Could you check a few things on this drawing? It's one solid part, dimensions in mm from its lowest x, y, z. A direction names the side the tool comes from. Round coordinates to 2 decimals unless told otherwise and drop trailing zeros. Write each loop counter-clockwise with the first axis right and the second up, starting at its lowest first coordinate (ties: lowest second). Pieces come first, ordered by that corner, then holes. Notation, with made-up numbers: (57, 81.25) -> (99, 81.25) arc R27 cw to (99, 108.25) -> close; hole circle Ø11 at (38.5, 54). An arc over 180 degrees is marked (long way). Answer as CSV lines item,"result".
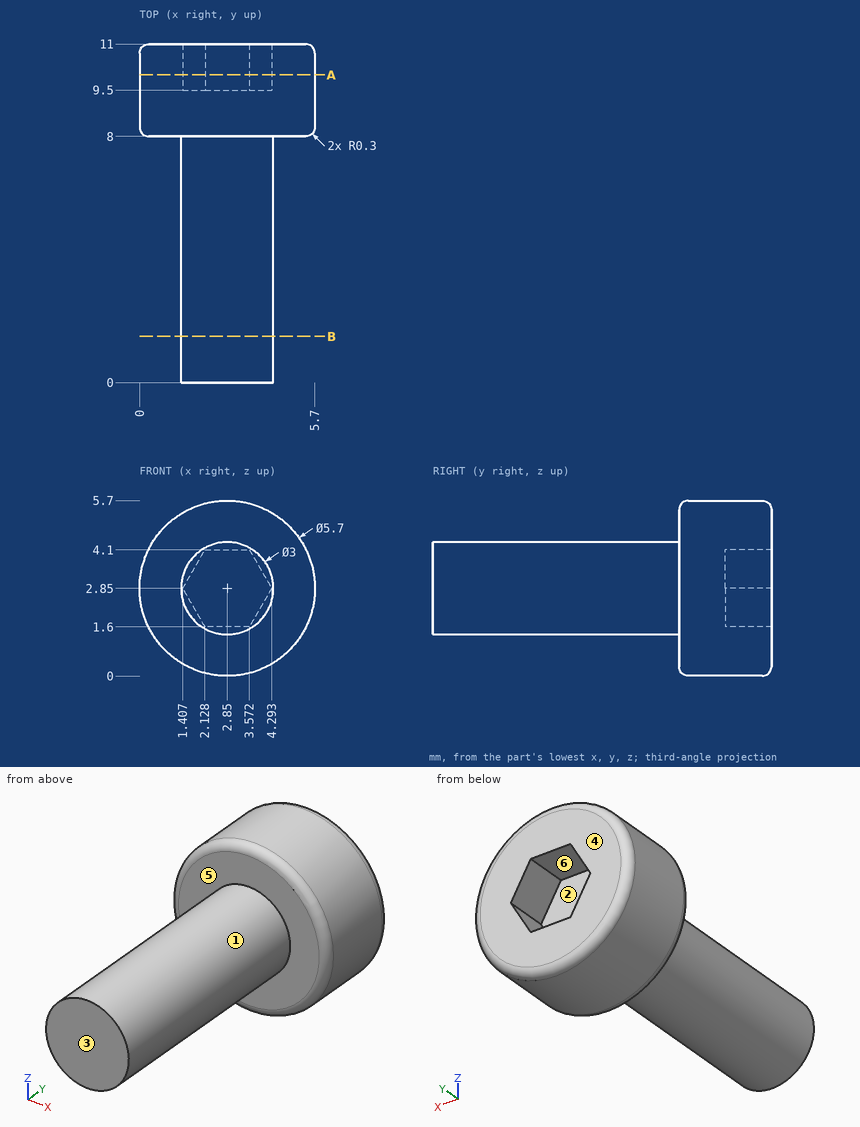
1. Suppose I cut it at A-A on y = 10. Please give me the cut outline in (x, z), and give its area (3 significant figures).
Numbers:
outline,"circle Ø5.7 at (2.85, 2.85); hole (1.41, 2.85) -> (2.13, 1.6) -> (3.57, 1.6) -> (4.29, 2.85) -> (3.57, 4.1) -> (2.13, 4.1) -> close"
area,"20.1 mm^2"
2. If we mould it in two halves opening along Z, with no side actions, what happens to the marked faces 1, 2 and 3? For each: released by +Z, released by -Z, zero draft, split by the parting line, or undercut.
Numbers:
face 1,"split by the parting line"
face 2,"undercut"
face 3,"zero draft"
3. If I drill on line 1 (Y direction, x = 1.65, z = 4.5); line 2 (Z direction, x = 3.2, y = 10.75) (1 decimal); line 3 (Y direction, x = 2.15, z = 2.05), over which ranges is the centre line in solid material (lowest first)?
Numbers:
line 1,"y = 8 to 11"
line 2,"z = 0 to 1.6, 4.1 to 5.7"
line 3,"y = 0 to 9.5"
4. Suppose I cut it at B-B on y = 1.5. Please give me the cut outline in (x, z).
Numbers:
outline,"circle Ø3 at (2.85, 2.85)"
5. For pin 1 Ø1 at (x, y) = (5, 9) entering from +Z; pin 2 Ø3 at (x, y) = (4, 4) entering from -Z, each with a flat end and sliding along its axis, tell me the tip position at first contact or that it passes through.
Numbers:
pin 1,"stops at z = 5.17"
pin 2,"stops at z = 1.35"
6. On a 3-axis mill with a long thin cutter (end or side, diameter ignored), from which of +Z, -Z, +X, -X, +Y, -Y can I reach the whole of each face in a straight line? I mean the marked faces 4, 5 and 6. Say none if no direction works.
Numbers:
face 4,"+Z, -Z, +X, -X, +Y"
face 5,"-Y"
face 6,"+Y"
